Could you check a few things on this model? Use its own coordinates, in mm. A direction names the side the tool comes from. Coordinates: 2 decimals unless noted, no trailing zeros. Loops run counter-clockwise (first coordinate to the right, second up) from the corner with the lowest first, then second, coordinate; pieces in that order, holes last. Notation, with made-up numbers: (-37, 15) -> (-25, 15) arc R21 ccw to (-25, 42) -> close; hole circle Ø11 at (54, 18.5). An arc over 180 degrees is marked (long way). One line per question, with ' | ' between items.
from build123d import *


with BuildPart() as f1:
    # F0 (on Top) → F1 (revolve)
    with BuildSketch(Plane.XY):
        Polygon((-6.49, 2.485), (-6.49, 0), (-6.49, -2.485), (-5.69, -2.485), (-5.69, -2.235), (-5.69, 0), (-5.69, 2.235), (-5.69, 2.485), align=None)
        Polygon((-3.875, 2.235), (-5.69, 2.235), (-5.69, 0), (-5.69, -2.235), (-3.875, -2.235), (-3.875, 0), align=None)
        Polygon((-3.875, 2.485), (-3.875, 2.235), (-3.875, 0), (-3.875, -2.235), (-3.875, -2.485), (-3.015, -2.485), (-3.015, 0), (-3.015, 2.485), align=None)
    revolve(axis=Axis((0, 2.798411, 0), (0, -1, 0)))


solid = f1.part
1) If we section it at B-B on z = 0: Please give me the cut outline in (x, y) (3 decimals), and give its area (3 significant figures).
Data:
outline: (-6.49, -2.485) -> (-5.69, -2.485) -> (-5.69, -2.235) -> (-3.875, -2.235) -> (-3.875, -2.485) -> (-3.015, -2.485) -> (-3.015, 2.485) -> (-3.875, 2.485) -> (-3.875, 2.235) -> (-5.69, 2.235) -> (-5.69, 2.485) -> (-6.49, 2.485) -> close; (3.015, -2.485) -> (3.875, -2.485) -> (3.875, -2.235) -> (5.69, -2.235) -> (5.69, -2.485) -> (6.49, -2.485) -> (6.49, 2.485) -> (5.69, 2.485) -> (5.69, 2.235) -> (3.875, 2.235) -> (3.875, 2.485) -> (3.015, 2.485) -> close | area: 32.7 mm²
2) We'd pull the mould along X, two halves only. Please class faces 1 (the face through (-6.19, -0.03, -1.95)), 2 (the face through (3, -2.485, 2)), 3 (the face through (-4, -2.235, 1)): pulls with the +X half, pulls with the -X half, needs draft (parallel to the pull), parting line crosses it, or undercut.
Data:
face 1: parting line crosses it | face 2: needs draft | face 3: undercut
3) If we section it at A-A on x = 0: Please give me the cut outline in (y, z) (3 decimals).
Data:
outline: (-2.485, -6.49) -> (2.485, -6.49) -> (2.485, -5.69) -> (2.235, -5.69) -> (2.235, -3.875) -> (2.485, -3.875) -> (2.485, -3.015) -> (-2.485, -3.015) -> (-2.485, -3.875) -> (-2.235, -3.875) -> (-2.235, -5.69) -> (-2.485, -5.69) -> close; (-2.485, 3.015) -> (2.485, 3.015) -> (2.485, 3.875) -> (2.235, 3.875) -> (2.235, 5.69) -> (2.485, 5.69) -> (2.485, 6.49) -> (-2.485, 6.49) -> (-2.485, 5.69) -> (-2.235, 5.69) -> (-2.235, 3.875) -> (-2.485, 3.875) -> close
4) If we section it at D-D on y = -0.1: Please give me the cut outline in (x, z) (3 decimals).
Data:
outline: circle Ø12.98 at (0, 0); hole circle Ø6.03 at (0, 0)
5) I'm going to push flat-ended pins straight in: pin 1 Ø1 at (x, z) = (-5, 1) entering from -Y (3 decimals); pin 2 Ø2 at (x, y) = (4, -1.5) entering from +Z (3 decimals); pin 3 Ø1 at (x, y) = (-3.5, 1) entering from -Z (3 decimals). Where does each tip first touch, or does it pass through?
Data:
pin 1: y = -2.235 | pin 2: z = 5.755 | pin 3: z = -5.755
6) If we section it at C-C on x = 4.75: Please give me the cut outline in (y, z) (3 decimals).
Data:
outline: (-2.485, -4.422) -> (2.485, -4.422) -> (2.485, -3.133) -> (2.235, -3.133) -> (2.235, 3.133) -> (2.485, 3.133) -> (2.485, 4.422) -> (-2.485, 4.422) -> (-2.485, 3.133) -> (-2.235, 3.133) -> (-2.235, -3.133) -> (-2.485, -3.133) -> close
7) I need wall thicknesses on line 1 along Z through (x, y) = (0, -2.4) (3 decimals); line 2 along X through (y, z) = (1, 0) (3 decimals). Which ranges of each line are inside material? Lowest first, please. Write a range as from..to.
Data:
line 1: -6.49..-5.69, -3.875..-3.015, 3.015..3.875, 5.69..6.49 | line 2: -6.49..-3.015, 3.015..6.49
8) On a 3-axis mill with a long thin cutter (end or side, diameter ignored), from which of +Z, -Z, +X, -X, +Y, -Y can I reach the whole of each face in a straight line? I mean faces 4 (the face through (4, 2.235, 1)), 5 (the face through (0, -2.485, 6)). Say none if no direction works.
Data:
face 4: +Y | face 5: +Z, -Z, +X, -X, -Y
